Design review of the part built by this model. Coordinates are the model's own, in mm. A direction names the side the tool comes from. Give positions to 0.01 mm unless a question says otherwise; leave off trailing zeros. Loops run counter-clockwise (first coordinate to the right, second up) from the corner with the lowest first, then second, coordinate; pieces in that order, holes last. Notation, with made-up numbers: (12.5, -20.75) -> (56.5, -20.75) arc R31 ccw to (56.5, 16.25) -> close; hole circle Ø6 at (82, -3.75). An arc over 180 degrees is marked (long way). Answer as CSV lines item,"result".
Autodesk Fusion 360 part; units mm, degrees
sketch "Sketch1" plane through (0, 0, 0) normal (1, 0, 0) x (0, 0, -1)
  circle A0 centre (0, 0) radius 2.5
  circle A1 centre (0, 0) radius 7.5
  line L0 (0, 0) -> (0, 40)
  circle A2 centre (0, 40) radius 5
  line L1 (-5, 40) -> (-7.4852, 0.4706)
  line L2 (5, 40) -> (7.4852, 0.4706)
  dimension "d1" = 5
  dimension "d2" = 5
  dimension "d3" = 40
  dimension "d4" = 10
  dimension "d5" = 39.5294
  dimension "d6" = 39.5294
extrude "Extrude1" add sketch "Sketch1" along normal mid plane 10 contours A1
extrude "Extrude2" add sketch "Sketch1" along normal mid plane 5 contours A1 L0 A2 L1 | A1 L0 A2 L2
extrude "Extrude3" add sketch "Sketch1" along normal mid plane 60 contours A2
Q1. We need section B-B, the plane x = -1. State the section outline as (y, z) points.
Filled sheet:
outline,"(0.47, -7.49) -> (40, -5) arc R5 ccw to (40, 5) -> (0.47, 7.49) arc R7.5 ccw (long way) to start; hole circle Ø5 at (0, 0)"
Q2. The part is to be moulded in two halves that separate along Y. For faces 1 (the flat face through (-5, 2, 2)), 2 (the flat face through (-0.035, 20.512, -6.225)), 3 (the cylindrical face through (-0.07, -7.436, 0.976)), say which applies: pulls with the +Y half, pulls with the -Y half, needs draft (parallel to the pull), parting line crosses it, or undercut.
Filled sheet:
face 1,"needs draft"
face 2,"pulls with the +Y half"
face 3,"undercut"
Q3. We need section A-A, the plane z = 0. State the section outline as (x, y) points, and give its area (4 significant figures).
Filled sheet:
outline,"(-30, 35) -> (-2.5, 35) -> (-2.5, 7.5) -> (-5, 7.5) -> (-5, 2.5) -> (5, 2.5) -> (5, 7.5) -> (2.5, 7.5) -> (2.5, 35) -> (30, 35) -> (30, 45) -> (-30, 45) -> close; (-5, -7.5) -> (5, -7.5) -> (5, -2.5) -> (-5, -2.5) -> close"
area,"837.5 mm^2"
Q4. Clearance check with flat-ended pins moving along their axes: pin 1 Ø1 at (y, z) = (32.5, -2.5) entering from +X; pin 2 Ø4 at (y, z) = (27.5, -4.5) entering from -X; pin 3 Ø4.5 at (y, z) = (3.5, 1.5) entering from -X. State where each tip first meets the part, or that it passes through.
Filled sheet:
pin 1,"stops at x = 2.5"
pin 2,"stops at x = -2.5"
pin 3,"stops at x = -5"
Q5. We need section C-C, the plane y = 39. State the section outline as (x, z) points, and give its area (3 significant figures).
Filled sheet:
outline,"(-30, -4.9) -> (-2.5, -4.9) -> (-2.5, -5.06) -> (2.5, -5.06) -> (2.5, -4.9) -> (30, -4.9) -> (30, 4.9) -> (2.5, 4.9) -> (2.5, 5.06) -> (-2.5, 5.06) -> (-2.5, 4.9) -> (-30, 4.9) -> close"
area,"590 mm^2"
Q6. For faces 4 (the flat face through (5, 2, 2)), 5 (the cylindrical face through (-0.42, 44.88, 1.08)), 6 (the cylindrical face through (0.07, -2.44, 0.54)), list the 3-axis set-ups (+Z, -Z, +X, -X, +Y, -Y) from which the entire face can be reached by the end or side of a thin tool; tool diameter is ignored.
Filled sheet:
face 4,"+Z, -Z, +X, -Y"
face 5,"none"
face 6,"+X, -X"
Q7. We need section D-D, the plane z = 4. State the section outline as (x, y) points.
Filled sheet:
outline,"(-30, 37) -> (-2.5, 37) -> (-2.5, 6.34) -> (-5, 6.34) -> (-5, -6.34) -> (5, -6.34) -> (5, 6.34) -> (2.5, 6.34) -> (2.5, 37) -> (30, 37) -> (30, 43) -> (-30, 43) -> close"
Q8. To check wall thickness, follow probe 1 along Z at (x, y) = (0, 0); probe 2 along Y at (x, z) = (2, 0); probe 3 along X at (y, z) = (16, -2). State the ranges of each line that lie inside material, in increasing order. Write a range as from..to.
Filled sheet:
probe 1,"z = -7.5..-2.5, 2.5..7.5"
probe 2,"y = -7.5..-2.5, 2.5..45"
probe 3,"x = -2.5..2.5"
